Verification items for the finished model (mm, model axes). A direction names the side the tool comes from. Give positions to 0.01 mm unless a question says otherwise; leave off trailing zeros. Loops run counter-clockwise (first coordinate to the right, second up) from the corner with the lowest first, then second, coordinate; pieces in that order, holes last. Notation, with made-up numbers: (-34.5, -31.75) -> (16.5, -31.75) arc R25 cw to (16.5, 5.25) -> close; hole circle Ø6 at (22.25, 7.25). An arc over 180 degrees is marked (long way). Answer in a Markdown table with one row per item. Add a question column.
Q1. Section check C-C on x = 27.5. Enter the section's corners in (y, z), and give its area (3 significant figures).
Q2. Material ranges on probe 1 along X at (y, z) = (-21.75, 37); probe 2 along Z at (x, y) = (21.5, -18.25), recorded low to high.
Q3. Set-up check for faces 1 (the face through (33.699, -13, 37)), 2 (the face through (41, -25.4, 22)): record each of +Z, -Z, +X, -X, +Y, -Y from which the full face is reachable in a straight line by a thin tool's end or side.
Q4. Gauge pin test, flat ends, axial feed: P1, Ø7.5, axis at y = -18.5, z = 36, coming from the -X side; P2, Ø12, axis at x = 9.5, y = -19, coming from the +Z side. Record the tip position at first contact, or that the pin passes through.
Q5. Section check B-B on z = 46. Enter the section's corners in (x, y).
```python
from build123d import *

# Parameters (mm, degrees)
F1_DEPTH  = 25.4
F1_FACE_W = 25.4
F1_FACE_H = 55.573448
F2_DEPTH  = 12.7


with BuildPart() as f1:
    # F0 (on Front) → F1 (new body)
    with BuildSketch(Plane.XZ):
        Polygon((0, 18.721553), (0, 0), (55.573452, 0), (55.573452, 55.573449), (33.698794, 55.573449), (33.698794, 18.721553), align=None)
    extrude(amount=F1_DEPTH)

    # F1_face (on face) → F2 (join, symmetric)
    with BuildSketch(Plane(origin=(55.573452, -12.7, 27.786724), x_dir=(0, 1, 0), z_dir=(1, 0, 0))):
        Rectangle(F1_FACE_W, F1_FACE_H)
    extrude(amount=F2_DEPTH, both=True)


solid = f1.part
```
Taken from the geometry:
| question | item | result |
|---|---|---|
| 1 | outline | (-25.4, 0) -> (0, 0) -> (0, 18.72) -> (-25.4, 18.72) -> close |
| 1 | area | 476 mm² |
| 2 | probe 1 | x = 33.7 to 68.27 |
| 2 | probe 2 | z = 0 to 18.72 |
| 3 | face 1 | +Z, -X, +Y, -Y |
| 3 | face 2 | +Z, -Z, +X, -X, -Y |
| 4 | P1 | stops at x = 33.7 |
| 4 | P2 | stops at z = 18.72 |
| 5 | outline | (33.7, -25.4) -> (68.27, -25.4) -> (68.27, 0) -> (33.7, 0) -> close |
